Here's how the part is built. I have some questions about the finished solid (model axes, mm). Face numbers are marked on the shaded views. A direction names the side the tool comes from. Coordinates: 2 decimals unless noted, no trailing zeros. Order: outer loops, then holes, each group sorted by start corner. A loop starts at its lowest first (then second) coordinate and runs counter-clockwise, first axis right, second up. Notation, with made-up numbers: M -2.5,-28.75 L 35.5,-28.75 A19 ccw 35.5,-20.75 Z; hole C -26,13 d7. An arc over 180 degrees is marked long. One line per question, with ' | ' between items. Start each with the question number.
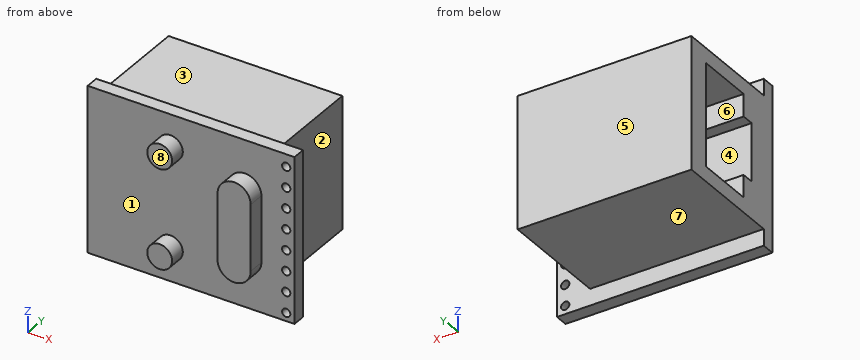
```python
from build123d import *

# Parameters (mm, degrees)
SKETCH1_W           = 25
SKETCH1_H           = 20
BOSS_EXTRUDE1_DEPTH = 1.6
SKETCH2_W           = 21
SKETCH2_H           = 16
BOSS_EXTRUDE2_DEPTH = 13.5
CUT_EXTRUDE1_DEPTH  = 13.5
SKETCH4_R           = 0.5
CUT_EXTRUDE2_DEPTH  = 13.5
BOSS_EXTRUDE3_DEPTH = 2
SKETCH6_R           = 1.5
BOSS_EXTRUDE4_DEPTH = 2


with BuildPart() as part:
    # Sketch1 → Boss-Extrude1 (new body)
    with BuildSketch(Plane(origin=(0, 0, 0), x_dir=(1, 0, 0), z_dir=(0, 1, 0))):
        Rectangle(SKETCH1_W, SKETCH1_H)
    extrude(amount=-BOSS_EXTRUDE1_DEPTH)

    # Sketch2 → Boss-Extrude2 (add)
    with BuildSketch(Plane(origin=(0, 0, 0), x_dir=(1, 0, 0), z_dir=(0, 1, 0))):
        with Locations((-2, 0)):
            Rectangle(SKETCH2_W, SKETCH2_H)
    extrude(amount=BOSS_EXTRUDE2_DEPTH)

    # Sketch3 → Cut-Extrude1 (cut)
    with BuildSketch(Plane.ZY.offset(12.5)):
        Polygon((-6.2, 3.75), (-3.5, 3.75), (-3.5, 2.25), (3.5, 2.25), (3.5, 3.75), (6.2, 3.75), (6.2, 10.75), (-6.2, 10.75), align=None)
    extrude(amount=-CUT_EXTRUDE1_DEPTH, mode=Mode.SUBTRACT)

    # Sketch4 → Cut-Extrude2 (cut)
    with BuildSketch(Plane(origin=(0, 0, 0), x_dir=(1, 0, 0), z_dir=(0, 1, 0))):
        with Locations(Location((11.5, 9, 0), (0, 0, 270))):
            Circle(SKETCH4_R)
        with Locations(Location((11.5, 6.5, 0), (0, 0, 270))):
            Circle(SKETCH4_R)
        with Locations(Location((11.5, 4, 0), (0, 0, 270))):
            Circle(SKETCH4_R)
        with Locations(Location((11.5, 1.5, 0), (0, 0, 270))):
            Circle(SKETCH4_R)
        with Locations(Location((11.5, -1, 0), (0, 0, 270))):
            Circle(SKETCH4_R)
        with Locations(Location((11.5, -3.5, 0), (0, 0, 270))):
            Circle(SKETCH4_R)
        with Locations(Location((11.5, -6, 0), (0, 0, 270))):
            Circle(SKETCH4_R)
        with Locations(Location((11.5, -8.5, 0), (0, 0, 270))):
            Circle(SKETCH4_R)
    extrude(amount=-CUT_EXTRUDE2_DEPTH, mode=Mode.SUBTRACT)

    # Sketch5 → Boss-Extrude3 (add)
    with BuildSketch(Plane(origin=(0, -1.6, 0), x_dir=(-1, 0, 0), z_dir=(0, -1, 0))):
        with BuildLine():
            Line((-8.5, -4), (-8.5, 4))
            ThreePointArc((-8.5, 4), (-6.5, 6), (-4.5, 4))
            Line((-4.5, 4), (-4.5, -4))
            ThreePointArc((-4.5, -4), (-6.5, -6), (-8.5, -4))
        make_face()
    extrude(amount=BOSS_EXTRUDE3_DEPTH)

    # Sketch6 → Boss-Extrude4 (add)
    with BuildSketch(Plane.XZ.offset(1.6)):
        with Locations(Location((-2.5, 6, 0), (0, 0, 270))):
            Circle(SKETCH6_R)
        with Locations(Location((-2.5, -6, 0), (0, 0, 270))):
            Circle(SKETCH6_R)
    extrude(amount=BOSS_EXTRUDE4_DEPTH)


solid = part.part
```
1. Imagine slicing it at C-C (y = 6). List the corners of the cut face in (x, z) for me, then the cut area to 3 significant figures.
2. I need wall thicknesses on line 1 (X direction, y = -1.3, z = -9); line 2 (Y direction, x = -11.25, z = -3.25); line 3 (Y direction, x = -8.5, z = -5.25). Which ranges of each line are inside material? Lowest first, please.
3. Imagine slicing it at D-D (x = 6.5). List the corners of the cut face in (y, z) for me.
4. Imagine slicing it at B-B (x = -2.5). List the corners of the cut face in (y, z) for me.
5. Imagine slicing it at A-A (z = -1.5). List the corners of the cut face in (x, y) for me, then the cut area to 3 significant figures.
6. We'd pull the mould along Z, two halves only. Please class the marked faces 6, 7 and 8: released by +Z, released by -Z, zero draft, split by the parting line, or undercut.
7. Which directions (+Z, -Z, +X, -X, +Y, -Y) give clear straight access to the entire face, cutting with the end or side of a thin tool? Please do the marked faces 1, 2, 3, 4 and 5.
8. Will these pins go through, and if not, where does the flat tip stop? pin 1 (10 mm diameter, centred on x = -2.5, z = -2, fed in from -Y); pin 2 (2.5 mm diameter, centred on y = 5, z = 1.5, fed in from -X); pin 3 (3 mm diameter, centred on y = 6, z = 7.5, fed in from +X); pin 4 (7 mm diameter, centred on x = -2.5, y = 4, fed in from -Z).
Entries:
1) outline: M -12.5,-8 L 8.5,-8 L 8.5,8 L -12.5,8 L -12.5,6.2 L 1,6.2 L 1,-6.2 L -12.5,-6.2 Z | area: 169 mm²
2) line 1: -12.5 to 11, 12 to 12.5 | line 2: -1.6 to 2.25, 10.75 to 13.5 | line 3: -1.6 to 3.75, 10.75 to 13.5
3) outline: M -3.6,-6 L -1.6,-6 L -1.6,-10 L 0,-10 L 0,-8 L 13.5,-8 L 13.5,8 L 0,8 L 0,10 L -1.6,10 L -1.6,6 L -3.6,6 Z
4) outline: M -3.6,-7.5 L -1.6,-7.5 L -1.6,-10 L 0,-10 L 0,-8 L 13.5,-8 L 13.5,8 L 0,8 L 0,10 L -1.6,10 L -1.6,7.5 L -3.6,7.5 L -3.6,4.5 L -1.6,4.5 L -1.6,-4.5 L -3.6,-4.5 Z; hole M 2.25,-3.5 L 3.75,-3.5 L 3.75,-6.2 L 10.75,-6.2 L 10.75,6.2 L 3.75,6.2 L 3.75,3.5 L 2.25,3.5 Z
5) outline: M -12.5,-1.6 L 4.5,-1.6 L 4.5,-3.6 L 8.5,-3.6 L 8.5,-1.6 L 11,-1.6 L 11,0 L 8.5,0 L 8.5,13.5 L -12.5,13.5 L -12.5,10.75 L 1,10.75 L 1,2.25 L -12.5,2.25 Z; M 12,-1.6 L 12.5,-1.6 L 12.5,0 L 12,0 Z | area: 215 mm²
6) face 6: undercut | face 7: released by -Z | face 8: zero draft
7) face 1: -Y | face 2: +Z, -Z, +X, +Y | face 3: +Z, +X, -X, +Y | face 4: -X | face 5: +Z, -Z, +X, -X, +Y
8) pin 1: y = -3.6 | pin 2: x = 1 | pin 3: x = 8.5 | pin 4: z = -8
